Here's how the part is built. I have some questions about the finished solid (model axes, mm). Round coordinates to 2 decimals unless told otherwise and drop trailing zeros. Write each loop counter-clockwise with the first axis right and the second up, starting at its lowest first coordinate (ties: lowest second). Pieces come first, ordered by that corner, then holes. Notation, with made-up numbers: (-26.75, 64) - (24.25, 64) arc R37 ccw to (24.25, 103) - close; hole circle Ø1 at (-24, -13.75). An arc over 180 degrees is marked (long way). Use one line per item in the form item = value. Start each with the question number.
1. Will this pin go through, and if not, where does the flat tip stop? pin 1 (1.2 mm diameter, centred on x = 10, y = -1, fed in from +Z).
2. If I drill on line 1 along X through (y, z) = (-0.9, 6.25); line 2 along X through (y, z) = (-4.15, 5.5); line 3 along Z through (x, y) = (10.25, -4.2), over which ranges is the centre line in solid material (lowest first)?
3. I want a section at B-B, the plane y = -4.3. List the corners of the cut face in (x, z) for me, plus the area to 3 significant figures.
4. I want a section at C-C, the plane z = 5.25. State how many separate pieces and enclosed holes the cut face has, plus the area to 4 significant figures.
5. I want a section at D-D, the plane y = -1.4. List the corners of the cut face in (x, z) for me, plus the area to 3 significant figures.
```python
from build123d import *

# Parameters (mm, degrees)
SKETCH2_W            = 10.41
SKETCH2_H            = 5
SKETCH2_W_2          = 1.7
SKETCH2_H_2          = 1
SKETCH2_W_3          = 2.2
SKETCH2_H_3          = 1.5
BOSS_EXTRUDE1_DEPTH  = 12
SKETCH3_W            = 2.2
SKETCH3_H            = 1.5
SKETCH3_W_2          = 1.7
SKETCH3_H_2          = 1.01
BOSS_EXTRUDE10_DEPTH = 5


with BuildPart() as part:
    # Sketch2 → Boss-Extrude1 (new body)
    with BuildSketch(Plane.XY):
        with Locations((6.39898523, -2.364078969)):
            Rectangle(SKETCH2_W, SKETCH2_H)
        with Locations((10.18198523, -4.354078969)):
            Rectangle(SKETCH2_W_2, SKETCH2_H_2, mode=Mode.SUBTRACT)
        with Locations((2.61598523, -4.354078969)):
            Rectangle(SKETCH2_W_2, SKETCH2_H_2, mode=Mode.SUBTRACT)
        with Locations((10.18198523, -1.114078969)):
            Rectangle(SKETCH2_W_3, SKETCH2_H_3, mode=Mode.SUBTRACT)
        with Locations((2.61598523, -1.114078969)):
            Rectangle(SKETCH2_W_3, SKETCH2_H_3, mode=Mode.SUBTRACT)
        with Locations((7.65998523, -1.114078969)):
            Rectangle(SKETCH2_W_3, SKETCH2_H_3, mode=Mode.SUBTRACT)
        with Locations((5.13798523, -1.114078969)):
            Rectangle(SKETCH2_W_3, SKETCH2_H_3, mode=Mode.SUBTRACT)
        with Locations((5.13798523, -4.354078969)):
            Rectangle(SKETCH2_W_2, SKETCH2_H_2, mode=Mode.SUBTRACT)
        with Locations((7.65998523, -4.354078969)):
            Rectangle(SKETCH2_W_2, SKETCH2_H_2, mode=Mode.SUBTRACT)
    extrude(amount=BOSS_EXTRUDE1_DEPTH)

    # Sketch3 → Boss-Extrude10 (add)
    with BuildSketch(Plane.XY):
        with Locations((10.18198523, -1.114078969)):
            Rectangle(SKETCH3_W, SKETCH3_H)
        with Locations((7.65998523, -1.114078969)):
            Rectangle(SKETCH3_W, SKETCH3_H)
        with Locations((5.13798523, -1.114078969)):
            Rectangle(SKETCH3_W, SKETCH3_H)
        with Locations((2.61598523, -1.114078969)):
            Rectangle(SKETCH3_W, SKETCH3_H)
        with Locations((5.13798523, -4.359078969)):
            Rectangle(SKETCH3_W_2, SKETCH3_H_2)
        with Locations((2.61598523, -4.359078969)):
            Rectangle(SKETCH3_W_2, SKETCH3_H_2)
        with Locations((7.65998523, -4.359078969)):
            Rectangle(SKETCH3_W_2, SKETCH3_H_2)
        with Locations((10.18198523, -4.359078969)):
            Rectangle(SKETCH3_W_2, SKETCH3_H_2)
    extrude(amount=BOSS_EXTRUDE10_DEPTH)


solid = part.part
```
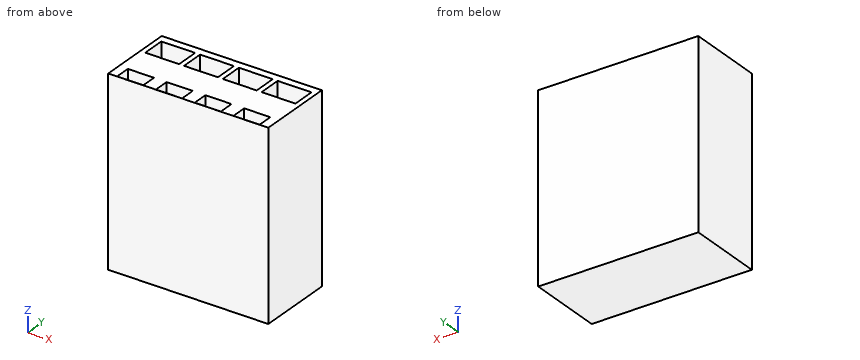
Model answer:
q1.pin_1 = 5
q2.line_1 = 1.19 to 1.52, 3.72 to 4.04, 6.24 to 6.56, 8.76 to 9.08, 11.28 to 11.6
q2.line_2 = 1.19 to 1.77, 3.47 to 4.29, 5.99 to 6.81, 8.51 to 9.33, 11.03 to 11.6
q2.line_3 = 0 to 5
q3.outline = (1.19, 0) - (11.6, 0) - (11.6, 12) - (11.03, 12) - (11.03, 5) - (9.33, 5) - (9.33, 12) - (8.51, 12) - (8.51, 5) - (6.81, 5) - (6.81, 12) - (5.99, 12) - (5.99, 5) - (4.29, 5) - (4.29, 12) - (3.47, 12) - (3.47, 5) - (1.77, 5) - (1.77, 12) - (1.19, 12) - close
q3.area = 77.3 mm2
q4.separate_pieces = 1
q4.enclosed_holes = 8
q4.area = 32.05 mm2
q5.outline = (1.19, 0) - (11.6, 0) - (11.6, 12) - (11.28, 12) - (11.28, 5) - (9.08, 5) - (9.08, 12) - (8.76, 12) - (8.76, 5) - (6.56, 5) - (6.56, 12) - (6.24, 12) - (6.24, 5) - (4.04, 5) - (4.04, 12) - (3.72, 12) - (3.72, 5) - (1.52, 5) - (1.52, 12) - (1.19, 12) - close
q5.area = 63.3 mm2
